from build123d import *

# Parameters (mm, degrees)
F0_W      = 71.755
F0_H      = 71.755
F1_DEPTH  = 7.874
F2_R      = 11.1125
F3_DEPTH  = 25.4
F5_D      = 5.1054
F7_R      = 33.3375
F8_DEPTH  = 19.1262
F9_R      = 4.7625
F10_DEPTH = 25.4
F6_R      = 29.36875
F11_DEPTH = 3.8862
F13_R     = 5.08


with BuildPart() as f1:
    # F0 (on Front) → F1 (new body)
    with BuildSketch(Plane.XZ):
        Rectangle(F0_W, F0_H)
    extrude(amount=-F1_DEPTH)

    # F2 (on face) → F3 (join)
    with BuildSketch(Plane.XZ):
        Circle(F2_R)
    extrude(amount=F3_DEPTH)

    # F5 (through all)
    with Locations(Plane.XZ):
        with Locations((27.6225, 27.6225), (27.6225, -27.6225), (-27.6225, -27.6225), (-27.6225, 27.6225)):
            Hole(F5_D / 2)

    # F7 (on face) → F8 (join)
    with BuildSketch(Plane(origin=(0, 7.874, 0), x_dir=(-1, 0, 0), z_dir=(0, 1, 0))):
        Circle(F7_R)
    extrude(amount=F8_DEPTH)

    # F9 (on face) → F10 (join)
    with BuildSketch(Plane(origin=(0, 27.0002, 0), x_dir=(-1, 0, 0), z_dir=(0, 1, 0))):
        with Locations((-23.8125, 0)):
            Circle(F9_R)
    extrude(amount=F10_DEPTH)

    # F6 (on face) → F11 (join)
    with BuildSketch(Plane.XZ):
        Circle(F6_R)
    extrude(amount=F11_DEPTH)

    # F12: F1 across plane


with BuildPart() as f1_1:
    add(f1.part)
    add(f1.part.mirror(Plane.YZ))

    # F13
    f13_edges = [f1_1.edges().sort_by_distance(p)[0] for p in [
        (35.8775, 3.937, 35.8775),
        (35.8775, 3.937, -35.8775),
        (-35.8775, 3.937, -35.8775),
        (-35.8775, 3.937, 35.8775),
    ]]
    fillet(f13_edges, radius=F13_R)


solid = f1_1.part
Read the model definition and answer for the solid it produces. Units are mm, in the model's axes. A direction names the side the tool comes from. Round coordinates to 2 decimals unless told otherwise and drop trailing zeros. Write each loop counter-clockwise with the first axis right and the second up, starting at its lowest first coordinate (ties: lowest second). Pieces come first, ordered by that corner, then holes.
Q1. Find section B-B on x = -27.5. Determine the outline of the cut face in (y, z), and give its area (3 significant figures).
Values:
outline: (-3.89, -10.31) - (0, -10.31) - (0, -25.07) - (7.87, -25.07) - (7.87, -18.85) - (27, -18.85) - (27, -3.01) - (52.4, -3.01) - (52.4, 3.01) - (27, 3.01) - (27, 18.85) - (7.87, 18.85) - (7.87, 25.07) - (0, 25.07) - (0, 10.31) - (-3.89, 10.31) - close; (0, -35.88) - (7.87, -35.88) - (7.87, -30.17) - (0, -30.17) - close; (0, 30.17) - (7.87, 30.17) - (7.87, 35.88) - (0, 35.88) - close
area: 1,440 mm2
Q2. Flat-ended cylindrical pins translate along their axes: P1, Ø5, axis at x = -19, z = -7.5, coming from the -Y side; P2, Ø3, axis at x = -27.62, z = -27.62, coming from the +Y side; P3, Ø6, axis at x = -16, y = 15, coming from the -Z side; P4, Ø8, axis at x = 27.62, z = -27.62, coming from the -Y side. Find the tip coordinate at first contact, or state that the pin passes through.
Values:
P1: stops at y = -3.89
P2: passes through
P3: stops at z = -30.7
P4: stops at y = 0
Q3. The mould has two halves that part along X. Classify faces 4 (the face through (28.57, 39.52, 0.21)), 5 (the face through (-31.8, 17.3, 10.01)), 6 (the face through (34.43, 3.99, -34.35)): released by +X, released by -X, zero draft, split by the parting line, or undercut.
Values:
face 4: undercut
face 5: split by the parting line
face 6: released by +X
Q4. Find section C-C on x = 0. Determine the outline of the cut face in (y, z), and give its area (3 significant figures).
Values:
outline: (-25.4, -11.11) - (-3.89, -11.11) - (-3.89, -29.37) - (0, -29.37) - (0, -35.88) - (7.87, -35.88) - (7.87, -33.34) - (27, -33.34) - (27, 33.34) - (7.87, 33.34) - (7.87, 35.88) - (0, 35.88) - (0, 29.37) - (-3.89, 29.37) - (-3.89, 11.11) - (-25.4, 11.11) - close
area: 2,550 mm2
Q5. A tool of negligible diameter and unlimited length cuts with its end or side. For faces 1 (the face through (-34.35, 3.99, 34.43)), 2 (the face through (-28.57, 39.52, 0.21)), 3 (the face through (10.6, -14.49, 3.34)), from which of +Z, -Z, +X, -X, +Y, -Y can it reach the whole face along a straight path? Write none if from no direction.
Values:
face 1: +Z, -X, +Y, -Y
face 2: +Y
face 3: -Y
Q6. Straight lines are drawn through the part: line 1 (Y direction, x = -6, z = -24.5); line 2 (Y direction, x = -2.5, z = -30); line 3 (Z direction, x = 5.5, y = -11.5). For each, find the intervals that lie inside material, in ascending order.
Values:
line 1: y = -3.89 to 27
line 2: y = 0 to 27
line 3: z = -9.66 to 9.66
